```python
from build123d import *

# Parameters (mm, degrees)
BOSS_EXTRUDE1_DEPTH = 9
CUT_EXTRUDE1_DEPTH  = 19
CUT_EXTRUDE2_DEPTH  = 10
CUT_EXTRUDE3_DEPTH  = 10
CUT_EXTRUDE4_DEPTH  = 10
CUT_EXTRUDE6_DEPTH  = 5


with BuildPart() as part:
    # Sketch1 → Boss-Extrude1 (new body)
    with BuildSketch(Plane.XY):
        Polygon((7.5, 1.5), (4.5, 4.5), (2.5, 4.5), (-1.5, 1.5), (-7.5, 1.5), (-7.5, -4.5), (7.5, -4.5), align=None)
    extrude(amount=BOSS_EXTRUDE1_DEPTH)

    # Sketch2 → Cut-Extrude1 (cut)
    with BuildSketch(Plane.ZY.offset(7.5)):
        Polygon((3, 4.5), (3, 3.5), (5, 3.5), (9, -4.5), (9, 4.5), align=None)
    extrude(amount=-CUT_EXTRUDE1_DEPTH, mode=Mode.SUBTRACT)

    # 3DSketch1 → Cut-Extrude2 (cut, along a direction that is not the sketch's normal)
    with BuildSketch(Plane(origin=(-7.5, 1.5, 0), x_dir=(0.4082482904638631, -0.816496580927726, 0.4082482904638631), z_dir=(0.7071067811865476, 0, -0.7071067811865476))):
        Polygon((0, 0), (4.898979486, 3.464101615), (7.348469228, 0), (0.816496581, -1.154700538), align=None)
    extrude(amount=-CUT_EXTRUDE2_DEPTH, dir=(1, 0, 0), mode=Mode.SUBTRACT)

    # 3DSketch2 → Cut-Extrude3 (cut, along a direction that is not the sketch's normal)
    with BuildSketch(Plane(origin=(-6.5, 1.5, 1), x_dir=(0.9352065538199315, -0.3359312898838437, 0.11197709662794787), z_dir=(0, -0.31622776601683794, -0.9486832980505139))):
        Polygon((0, 0), (4.10995504, 5.206560243), (5.045161594, 4.852457572), (8.930397645, 0), (4.676032769, -1.770513356), align=None)
    extrude(amount=-CUT_EXTRUDE3_DEPTH, dir=(0, 0, -1), mode=Mode.SUBTRACT)


with BuildPart() as body_2:
    # of the pieces the cut leaves, the one that is kept (cut_extrude3_keep)
    add(part.part.solids().sort_by_distance((7.5, 1.5, 0))[0])

    # 3DSketch3 → Cut-Extrude4 (cut, along a direction that is not the sketch's normal)
    with BuildSketch(Plane(origin=(7.5, 1.5, 1), x_dir=(-0.22453265936457553, -0.9244601540308832, 0.3081533846769612), z_dir=(0, 0.316227766016838, 0.9486832980505139))):
        Polygon((0, 0), (6.163067694, 1.420069225), (6.490274323, 0), align=None)
    extrude(amount=CUT_EXTRUDE4_DEPTH, dir=(0, 0, 1), mode=Mode.SUBTRACT)

    # Sketch4 → Cut-Extrude6 (cut)
    with BuildSketch(Plane.XY.offset(10)):
        Polygon((1.851766406, -4.5), (1.851766406, -1.5), (-3.5, -4.5), align=None)
    extrude(amount=-CUT_EXTRUDE6_DEPTH, mode=Mode.SUBTRACT)


solid = body_2.part
```
The listing builds one solid part. Answer for the finished solid, in the listing's coordinates (mm). A direction names the side the tool comes from. Coordinates: 2 decimals unless noted, no trailing zeros. Loops run counter-clockwise (first coordinate to the right, second up) from the corner with the lowest first, then second, coordinate; pieces in that order, holes last. Notation, with made-up numbers: M -20,68.5 L 16,68.5 A21 ccw 16,90.5 Z; hole C 20.5,9.5 d11. An arc over 180 degrees is marked long. Answer as a JSON object with one key per item and string values. Group by question number.
Item 1: Section D-D (x = -6) is taken. Write down the section's boundary in (y, z).
Item 2: Section C-C (y = -1.25) is taken. Write down the section's boundary in (x, z) (3 decimals), and give its area (3 significant figures).
Item 3: Each of these flat-tipped pins is pushed along its axis until it touches: P1, Ø0.9, axis at y = -3.5, z = 7, coming from the -X side; P2, Ø1.1, axis at x = -4.5, z = 0.5, coming from the +Y side; P3, Ø3, axis at x = -5.5, y = 0, coming from the +Z side. Where does it stop, or does it pass through?
Item 4: Section A-A (x = 4) is taken. Write down the section's boundary in (y, z), and give its area (3 significant figures).
Item 5: Determine the mould class of faces 6 (the face through (-0.84, -3.01, 3.65)), 7 (the face through (2, -4.5, 3)), 8 (the face through (4, 4.5, 1)), 9 (the face through (-6.4, -1.9, 1.1)) for opening direction Y: +Y half, -Y half, draft (parallel to the pull), parting line (faces both ways), or undercut.
Item 6: Consider L1, parallel to Y at x = 0.25, z = 3; L2, parallel to Y at x = 0.5, z = 0.75; L3, parallel to Y at x = -0.25, z = 4. Determine where each line is inside the solid, lowest interval first.
Item 7: Section B-B (z = 3.5) is taken. Write down the section's boundary in (x, y), and give its area (3 significant figures).
Item 8: Which of the six approach directions +Z, -Z, +X, -X, +Y, -Y give full straight-line access (tool end or side, diameter ignored) to faces 1 (the face through (3, 3.5, 4)), 2 (the face through (-2.6, -0.9, 1.8)), 3 (the face through (6.755, -1.566, 4.98)), 4 (the face through (-4.5, 1.5, 0.5)), 5 (the face through (1.852, -3, 7))?
Solved:
{
 "1": {"outline": "M -4.5,0 L 1.5,0 L 1.5,1 L 0,1.5 L -4.5,1.5 Z"},
 "2": {"outline": "M -7.5,0 L 7.5,0 L 7.5,1.917 L 6.832,1.917 L 6.832,7.375 L 1.572,7.375 L 1.572,1.917 L -5.583,1.917 Z", "area": "55.6 mm2"},
 "3": {"P1": "stops at x = 1.85", "P2": "stops at y = 1.5", "P3": "stops at z = 2"},
 "4": {"outline": "M -4.5,0 L 4.5,0 L 4.5,3 L 3.5,3 L 3.5,5 L -4.5,9 Z", "area": "59.0 mm2"},
 "5": {"face 6": "undercut", "face 7": "-Y half", "face 8": "+Y half", "face 9": "draft"},
 "6": {"L1": "y = -4.5 to -2.4, -0.07 to 2.81", "L2": "y = -4.5 to 3", "L3": "y = -4.5 to -2.68, 0.38 to 2.44"},
 "7": {"outline": "M -3.5,-4.5 L 6.04,-4.5 L 7.5,1.5 L 5.5,3.5 L 1.17,3.5 L -1.5,1.5 L 1.85,-1.5 Z", "area": "55.9 mm2"},
 "8": {"face 1": "+Z, +X, -X, +Y", "face 2": "+Z, -X", "face 3": "+Z, +X", "face 4": "+Z, -Z, -X, +Y", "face 5": "+Z, -X, -Y"}
}
